Can you work these out from the drawing? Everything is in mm from the part's minimum corner. Coordinates: 2 decimals unless noted, no trailing zeros. Loops run counter-clockwise (first coordinate to the right, second up) from the corner with the lowest first, then second, coordinate; pieces in that order, holes last. Notation, with made-up numbers: (44.5, 30.5) -> (84.5, 30.5) arc R20 cw to (84.5, 64.5) -> close; hole circle Ø7 at (18, -19.5). An arc over 180 degrees is marked (long way). Put each result on its own line as item: value. Start each with the question number.
Item 1: If we section it at A-A on x = 457.2: Please give me the cut outline in (y, z), plus the area to 3 significant figures.
Item 2: Please list where these lines run through material, in increasing order: L1, parallel to Y at x = 457.2, z = 9; L2, parallel to X at y = 672, z = 6; L3, parallel to Y at x = 386, z = 15. Write a range as from..to.
Item 3: If we section it at C-C on z = 17.25: State how many separate pieces and enclosed holes the cut face has, plus the area to 3 significant figures.
Item 4: If we section it at B-B on y = 391: Please give me the cut outline in (x, z), plus the area to 3 significant figures.
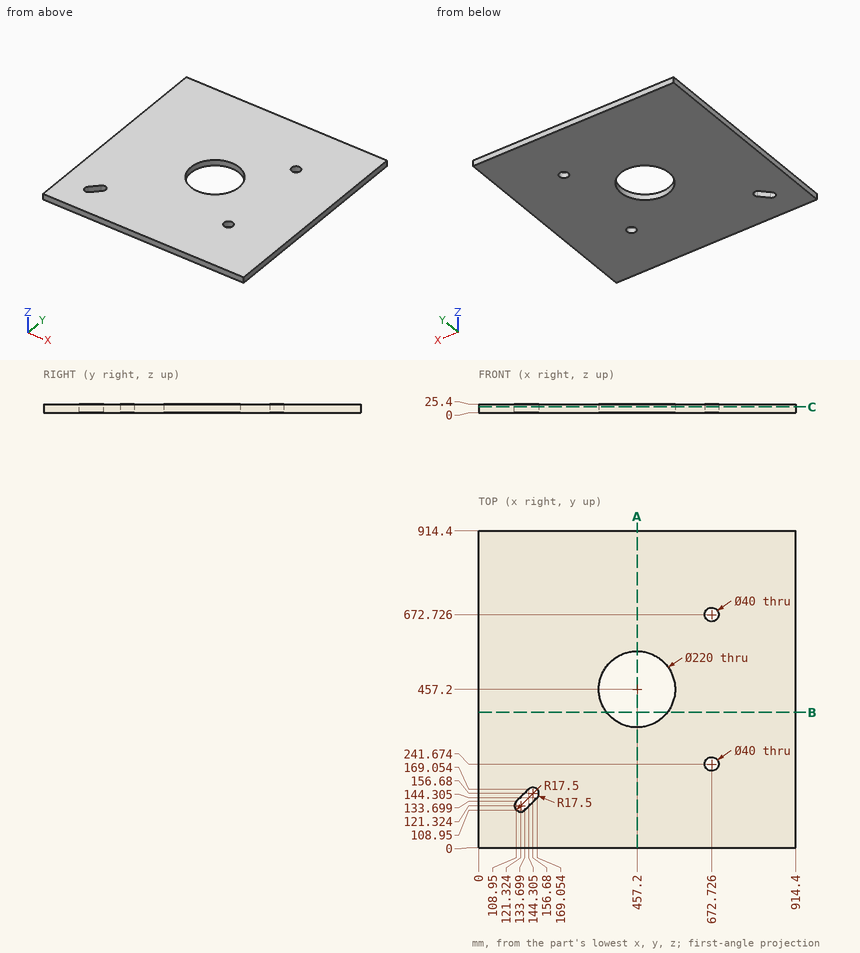
Solutions:
1. outline: (0, 0) -> (347.2, 0) -> (347.2, 25.4) -> (0, 25.4) -> close; (567.2, 0) -> (914.4, 0) -> (914.4, 25.4) -> (567.2, 25.4) -> close
1. area: 17,600 mm^2
2. L1: 0..347.2, 567.2..914.4
2. L2: 0..652.74, 692.71..914.4
2. L3: 0..373.35, 541.05..914.4
3. separate pieces: 1
3. enclosed holes: 4
3. area: 793,000 mm^2
4. outline: (0, 0) -> (369.35, 0) -> (369.35, 25.4) -> (0, 25.4) -> close; (545.05, 0) -> (914.4, 0) -> (914.4, 25.4) -> (545.05, 25.4) -> close
4. area: 18,800 mm^2
